Work out the finished part from the listing and answer in its coordinate system (mm). Round coordinates to 2 decimals unless told otherwise and drop trailing zeros. Order: outer loops, then holes, each group sorted by start corner. A loop starts at its lowest first (then second) coordinate and runs counter-clockwise, first axis right, second up.
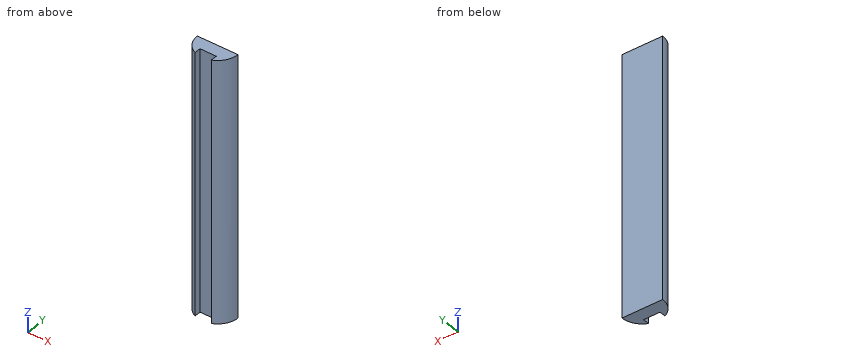
Autodesk Inventor part; units mm, degrees
ref_plane "YZ Plane" through (0, 0, 0) normal (1, 0, 0) x (0, 1, 0)
ref_plane "XZ Plane" through (0, 0, 0) normal (0, 1, 0) x (-1, 0, 0)
ref_plane "XY Plane" through (0, 0, 0) normal (0, 0, 1) x (1, 0, 0)
sketch "Sketch1" plane through (0, 0, 0) normal (0, 0, 1) x (1, 0, 0)
  line L0 (1.5575, -2.3616) -> (1.5482, -3.6067)
  line L1 (-1.5924, -2.3382) -> (1.5575, -2.3616)
  line L2 (-1.6017, -3.5833) -> (-1.5924, -2.3382)
  arc A0 (-1.5482, 3.6067) -> (-1.6017, -3.5833) centre (0, 0) ccw
  line L3 (-1.5575, 2.3616) -> (-1.5482, 3.6067)
  line L4 (1.5924, 2.3382) -> (-1.5575, 2.3616)
  line L5 (1.6017, 3.5833) -> (1.5924, 2.3382)
  arc A1 (1.5482, -3.6067) -> (1.6017, 3.5833) centre (0, 0) ccw
  point P0 (0, 0)
extrude "Extrusion1" add sketch "Sketch1" along normal blind 50
sketch "Sketch2" plane through (0, 0, 0) normal (0, 0, -1) x (-1, 0, 0)
  line L0 (-25, 13) -> (13, 13)
  line L1 (13, 13) -> (13, 0)
  line L2 (13, 0) -> (-25, 0)
  line L3 (-25, 0) -> (-25, 13)
  point P0 (0, 0)
extrude "Extrusion2" cut sketch "Sketch2" against normal blind 89.5
properties part number "Long_axel"
Item 1: Find the intervals of material crossed by line 1 along Y through (x, z) = (0.5, 5.5); line 2 along X through (y, z) = (-3.05, 17.5); line 3 along X through (y, z) = (-3.1, 5.5), in increasing order.
Item 2: Find section C-C (x = -3.5). Write down the section's boundary in (y, z), plus the area to 3 significant figures.
Item 3: Find section B-B (z = 13.5). Write down the section's boundary in (x, y), plus the area to 3 significant figures.
Item 4: Find section D-D (y = -1.1). Write down the section's boundary in (x, z).
Item 5: Find section A-A (y = -3). Write down the section's boundary in (x, z).
Model answer:
1. line 1: y = -2.35 to 0
1. line 2: x = -2.47 to -1.6, 1.55 to 2.47
1. line 3: x = -2.41 to -1.6, 1.55 to 2.41
2. outline: (-1.78, 0) - (0, 0) - (0, 50) - (-1.78, 50) - close
2. area: 88.8 mm2
3. outline: (-3.92, 0) arc R3.92 ccw to (-1.6, -3.58) - (-1.59, -2.34) - (1.56, -2.36) - (1.55, -3.61) arc R3.92 ccw to (3.92, 0) - close
3. area: 19.6 mm2
4. outline: (-3.77, 0) - (3.77, 0) - (3.77, 50) - (-3.77, 50) - close
5. outline: (-2.53, 0) - (-1.6, 0) - (-1.6, 50) - (-2.53, 50) - close; (1.55, 0) - (2.53, 0) - (2.53, 50) - (1.55, 50) - close
